from build123d import *

# Parameters (mm, degrees)
SKETCH2_W             = 374.0912
SKETCH2_H             = 117.5004
SKETCH2_R             = 16.25
SKETCH2_W_2           = 71.6
SKETCH2_H_2           = 23.6
BOSS_EXTRUDE1_DEPTH   = 4.191
F_4_40_TAPPED_HOLE1_D = 2.2606
SKETCH7_R             = 3.6449
SKETCH7_R_2           = 6.2484
SKETCH7_R_3           = 1.4986
SKETCH7_R_4           = 7
SKETCH7_R_5           = 5.7531
CUT_EXTRUDE1_DEPTH    = 393.132801993


with BuildPart() as part:
    # Sketch2 → Boss-Extrude1 (new body)
    with BuildSketch(Plane.XY):
        with Locations((187.0456, 58.7502)):
            Rectangle(SKETCH2_W, SKETCH2_H)
        with Locations((137.16, 34.9504)):
            Circle(SKETCH2_R, mode=Mode.SUBTRACT)
        with Locations((137.4, 80.3004)):
            Rectangle(SKETCH2_W_2, SKETCH2_H_2, mode=Mode.SUBTRACT)
    extrude(amount=BOSS_EXTRUDE1_DEPTH)

    # #4-40 Tapped Hole1 (through all)
    with Locations(Plane.XY.offset(4.191)):
        with Locations((99.9, 94.3004), (174.9, 94.3004), (174.9, 66.3004), (99.9, 66.3004)):
            Hole(F_4_40_TAPPED_HOLE1_D / 2)

    # Sketch7 → Cut-Extrude1 (cut, through all)
    with BuildSketch(Plane.XY.offset(4.191)):
        with Locations((211.3, 79.4004)):
            Circle(SKETCH7_R)
        with Locations((211.3, 56.5404)):
            Circle(SKETCH7_R_2)
        with Locations((211.3, 47.5488)):
            Circle(SKETCH7_R_3)
        with Locations((243.05, 79.4004)):
            Circle(SKETCH7_R)
        with Locations((243.05, 56.5404)):
            Circle(SKETCH7_R_2)
        with Locations((243.05, 47.5488)):
            Circle(SKETCH7_R_3)
        with Locations((274.8, 79.4004)):
            Circle(SKETCH7_R)
        with Locations((306.55, 79.4004)):
            Circle(SKETCH7_R)
        with Locations((306.55, 56.5404)):
            Circle(SKETCH7_R_2)
        with Locations((306.55, 47.5488)):
            Circle(SKETCH7_R_3)
        with Locations((344.65, 79.4004)):
            Circle(SKETCH7_R_4)
        with Locations((344.65, 56.5404)):
            Circle(SKETCH7_R_5)
        with BuildLine():
            Line((266.291, 52.288251097), (266.291, 60.792548903))
            ThreePointArc((266.291, 60.792548903), (274.8, 66.0527), (283.309, 60.792548903))
            Line((283.309, 60.792548903), (283.309, 52.288251097))
            ThreePointArc((283.309, 52.288251097), (274.8, 47.0281), (266.291, 52.288251097))
        make_face()
    extrude(amount=-CUT_EXTRUDE1_DEPTH, mode=Mode.SUBTRACT)


solid = part.part
Read the model definition and answer for the solid it produces. Units are mm, in the model's axes. Round coordinates to 2 decimals unless told otherwise and drop trailing zeros. Write each loop counter-clockwise with the first axis right and the second up, starting at its lowest first coordinate (ties: lowest second). Pieces come first, ordered by that corner, then holes.
1. The part is cut by section A-A, the plane x = 274.8. Determine the outline of the cut face in (y, z), then the cut area to 3 significant figures.
2. The part is cut by section B-B, the plane y = 28. Determine the outline of the cut face in (x, z), then the cut area to 3 significant figures.
3. Straight lines are drawn through the part: L1, parallel to X at y = 57, z = 0.9; L2, parallel to Y at x = 344.65, z = 2.8; L3, parallel to Y at x = 174.9, z = 2.9. For each, find the intervals that lie inside material, in ascending order.
4. Given pin 1 Ø2 at (x, z) = (126.5, 1.5) entering from -Y, flat-ended and moving along its own axis, determine where the tip first touches the part or whether it passes through.
5. The part is cut by section C-C, the plane z = 2. State how many separate pieces and enclosed holes the cut face has, then the cut area to 3 significant figures.
6. The part is cut by section D-D, the plane x = 137.16. Determine the outline of the cut face in (y, z).
7. Determine the mould class of faces 1 (the face through (214.777, 80.495, 2.125)), 2 (the face through (184, 60, 0)), 3 (the face through (184, 60, 4.191)) for opening direction Z: pulls with the +Z half, pulls with the -Z half, needs draft (parallel to the pull), parting line crosses it, or undercut.
Values:
1. outline: (0, 0) - (47.03, 0) - (47.03, 4.19) - (0, 4.19) - close; (66.05, 0) - (75.76, 0) - (75.76, 4.19) - (66.05, 4.19) - close; (83.05, 0) - (117.5, 0) - (117.5, 4.19) - (83.05, 4.19) - close
1. area: 382 mm2
2. outline: (0, 0) - (122.47, 0) - (122.47, 4.19) - (0, 4.19) - close; (151.85, 0) - (374.09, 0) - (374.09, 4.19) - (151.85, 4.19) - close
2. area: 1,440 mm2
3. L1: x = 0 to 205.07, 217.53 to 236.82, 249.28 to 266.29, 283.31 to 300.32, 312.78 to 338.92, 350.38 to 374.09
3. L2: y = 0 to 50.79, 62.29 to 72.4, 86.4 to 117.5
3. L3: y = 0 to 65.17, 67.43 to 93.17, 95.43 to 117.5
4. pin 1: stops at y = 0
5. separate pieces: 1
5. enclosed holes: 19
5. area: 40,300 mm2
6. outline: (0, 0) - (18.7, 0) - (18.7, 4.19) - (0, 4.19) - close; (51.2, 0) - (68.5, 0) - (68.5, 4.19) - (51.2, 4.19) - close; (92.1, 0) - (117.5, 0) - (117.5, 4.19) - (92.1, 4.19) - close
7. face 1: needs draft
7. face 2: pulls with the -Z half
7. face 3: pulls with the +Z half
